Solid Edge part; units mm, degrees
sketch "Sketch1" plane through (0, 0, 0) normal (0, 0, 1) x (1, 0, 0)
  line L0 (0, 24) -> (0, 16)
  line L1 (0, 16) -> (-6, 16)
  line L2 (-6, 16) -> (-16.7217, 5.2783)
  line L3 (-16.7217, 5.2783) -> (-16.7217, -5.2783)
  line L4 (-16.7217, -5.2783) -> (-6, -16)
  line L5 (-6, -16) -> (0, -16)
  line L6 (0, -16) -> (0, -24)
  line L7 (0, -24) -> (-6.4853, -24)
  line L8 (-6.4853, -24) -> (-25, -5.4853)
  line L9 (-25, -5.4853) -> (-25, 5.4853)
  line L10 (-25, 5.4853) -> (-6.4853, 24)
  line L11 (-6.4853, 24) -> (0, 24)
extrude "Protrusion1" add sketch "Sketch1" along normal mid plane 6
sketch "Sketch2" plane through (0, 0, 0) normal (0, 0, 1) x (1, 0, 0)
  line L0 (-6, -16) -> (0, -16)
  line L1 (0, -16) -> (0, -31)
  line L2 (0, -31) -> (-6, -31)
  line L3 (-6, -31) -> (-6, -16)
extrude "ExtrudedProtrusion_2" add sketch "Sketch2" along normal mid plane 6
sketch "Sketch3" plane through (-12.2288, -3.5, -3) normal (0, 0, -1) x (0, 1, 0)
  line L0 (8.7783, -4.4929) -> (8.7783, -12.7712)
  line L1 (8.7783, -12.7712) -> (8.9853, -12.7712)
  line L2 (8.9853, -12.7712) -> (27.5, 5.7435)
  line L3 (27.5, 5.7435) -> (27.5, 12.2288)
  line L4 (27.5, 12.2288) -> (19.5, 12.2288)
  line L5 (19.5, 12.2288) -> (19.5, 6.2288)
  line L6 (19.5, 6.2288) -> (8.7783, -4.4929)
extrude "Cutout1" cut sketch "Sketch3" against normal through all
sketch "Sketch4" plane through (0, 0, 0) normal (0, 0, 1) x (1, 0, 0)
  line L0 (-16.7217, 5.2783) -> (-25, 5.2783)
  line L1 (-25, 5.2783) -> (-25, 15.2783)
  line L2 (-25, 15.2783) -> (-10, 30.2783)
  line L3 (-10, 30.2783) -> (-10, 35.2783)
  line L4 (-10, 35.2783) -> (-5, 35.2783)
  line L5 (-5, 35.2783) -> (-5, 10.2783)
  line L6 (-5, 10.2783) -> (-16.7217, 10.2783)
  line L7 (-16.7217, 10.2783) -> (-16.7217, 5.2783)
  dimension "D1" = 16.7217
  dimension "D2" = 25
  dimension "D3" = 10
extrude "ExtrudedProtrusion_3" add sketch "Sketch4" along normal mid plane 6
hole "Hole_1" at (-11, 16.2783, -3) direction (0, 0, 1) diameter 5 end up to next
properties material "Polyethylene, low density"
Geometry check sheet. Reference: the model listing, model coordinates, mm. A direction names the side the tool comes from. Coordinates: 2 decimals unless noted, no trailing zeros. Order: outer loops, then holes, each group sorted by start corner. A loop starts at its lowest first (then second) coordinate and runs counter-clockwise, first axis right, second up.
Q1. Thickness scan on probe 1 along Y at (x, z) = (-11, 1.7); probe 2 along Y at (x, z) = (-9.75, -0.95); probe 3 along X at (y, z) = (5, 2.5). Record the ranges inside material, lowest first.
Reply:
probe 1: y = -19.49 to -11, 10.28 to 13.78, 18.78 to 29.28
probe 2: y = -20.74 to -12.25, 10.28 to 14.11, 18.44 to 35.28
probe 3: x = -25 to -16.72
Q2. Sectioned sample at D-D on x = -19.5. Record the cut outline in (y, z).
Reply:
outline: (-10.99, -3) - (20.78, -3) - (20.78, 3) - (-10.99, 3) - close
Q3. Depth check by flat-ended pin: pin 1 Ø3 at (x, z) = (-2.5, 1.5) entering from +Y; pin 2 Ø3 at (y, z) = (2, 0) entering from +X; pin 3 Ø1.8 at (y, z) = (25.5, 0) entering from +X; pin 4 Ø3 at (x, y) = (-18.5, 25.5) entering from -Z. Enter the tip coordinate at first touch or a pass-through.
Reply:
pin 1: stops at y = -16
pin 2: stops at x = -16.72
pin 3: stops at x = -5
pin 4: passes through
Q4. Sectioned sample at A-A on z = 0.1. Record the cut outline in (x, y).
Reply:
outline: (-25, -5.49) - (-6.49, -24) - (-6, -24) - (-6, -31) - (0, -31) - (0, -16) - (-6, -16) - (-16.72, -5.28) - (-16.72, 10.28) - (-5, 10.28) - (-5, 35.28) - (-10, 35.28) - (-10, 30.28) - (-25, 15.28) - close; hole circle Ø5 at (-11, 16.28)
Q5. Sectioned sample at B-B on x = -11. Record the cut outline in (y, z), and give its area (3 significant figures).
Reply:
outline: (-19.49, -3) - (-11, -3) - (-11, 3) - (-19.49, 3) - close; (10.28, -3) - (13.78, -3) - (13.78, 3) - (10.28, 3) - close; (18.78, -3) - (29.28, -3) - (29.28, 3) - (18.78, 3) - close
area: 135 mm2
Q6. Tool access check on faces 4 (the face through (-5, 23, 0)), 5 (the face through (-11, 10.278, 0)), 6 (the face through (-6, -28, 0)). Record the directions out of +Z, -Z, +X, -X, +Y, -Y that give a thin tool (end or side, any length) a straight path to the whole face; none if there is none.
Reply:
face 4: +Z, -Z, +X, +Y
face 5: +Z, -Z, +X
face 6: +Z, -Z, -X, -Y
Q7. Sectioned sample at C-C on y = 13. Record the cut outline in (x, z).
Reply:
outline: (-25, -3) - (-5, -3) - (-5, 3) - (-25, 3) - close
Q8. Draft check along X on faces 1 (the face through (-11, -11, 0)), 2 (the face through (-12.521, 14.294, -0.042)), 3 (the face through (-18, 2, -3)). Enter one of: released by +X, released by -X, zero draft, split by the parting line, or undercut.
Reply:
face 1: released by +X
face 2: undercut
face 3: zero draft
